Here's how the part is built. I have some questions about the finished solid (model axes, mm). Face numbers are marked on the shaded views. A direction names the side the tool comes from. Coordinates: 2 decimals unless noted, no trailing zeros. Write each loop counter-clockwise with the first axis right and the second up, starting at its lowest first coordinate (ties: lowest second). Pieces come first, ordered by that corner, then holes. Notation, with made-up numbers: (83.25, 34.25) -> (101.25, 34.25) arc R19 ccw to (101.25, 67.25) -> close; hole circle Ø10 at (-33.75, 5). An arc over 180 degrees is marked (long way). Use a Markdown table: item, result. Add a question column.
Item 1: If I drill on line 1 along Z through (x, y) = (6, -0.75); line 2 along Y through (x, z) = (-16.5, -3.5); line 3 along Y through (x, z) = (-10, -4.25), over which ranges is the centre line in solid material (lowest first)? Write a range as from..to.
Item 2: If we mould it in two halves opening along Z, with no side actions, what happens to the marked faces 1, 2 and 3? For each: pulls with the +Z half, pulls with the -Z half, needs draft (parallel to the pull), parting line crosses it, or undercut.
Item 3: Imagine slicing it at C-C, the plane x = 8.89. Write out the boundary of the cut face in (y, z).
Item 4: On a 3-axis mill with a long thin cutter (end or side, diameter ignored), from which of +Z, -Z, +X, -X, +Y, -Y can I reach the whole of each face in a straight line? I mean the marked faces 4, 5, 6, 7 and 8. Say none if no direction works.
Item 5: Imagine slicing it at D-D, the plane y = 8.75. Write out the boundary of the cut face in (x, z) (3 decimals), and give its area (3 significant figures).
Item 6: Will these pins go through, and if not, where does the flat tip stop? pin 1 Ø2 at (x, z) = (-2.5, 6.5) entering from -Y; pin 2 Ø5 at (y, z) = (6.5, -0.5) entering from +X; pin 3 Ø4 at (x, z) = (-3, -2) entering from -Y.
Item 7: Imagine slicing it at A-A, the plane y = 4.75. Write out the boundary of the cut face in (x, z) (3 decimals), and give its area (3 significant figures).
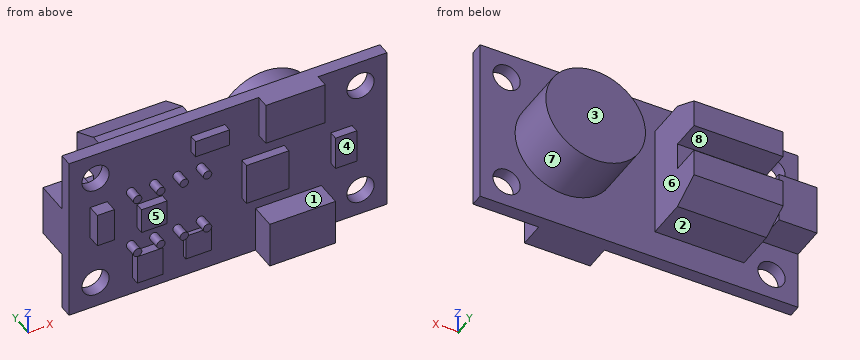
```python
from build123d import *

# Parameters (mm, degrees)
SKETCH1_W               = 38.1
SKETCH1_H               = 20.32
BOSS_EXTRUDE1_DEPTH     = 1.524
F_4_CLEARANCE_HOLE1_D   = 3.2639
SKETCH4_W               = 4.572
SKETCH4_H               = 6.096
BOSS_EXTRUDE2_DEPTH     = 4.064
SKETCH5_R               = 5.969
BOSS_EXTRUDE3_DEPTH     = 6.604
SKETCH6_W               = 10.668
SKETCH6_H               = 13.462
BOSS_EXTRUDE4_DEPTH     = 4.826
BOSS_EXTRUDE5_DEPTH     = 10.668
SKETCH8_W               = 7.874
SKETCH8_H               = 5.588
BOSS_EXTRUDE6_DEPTH     = 3.048
SKETCH9_W               = 7.112
SKETCH9_H               = 5.08
BOSS_EXTRUDE7_DEPTH     = 1.524
SKETCH10_W              = 2.54
SKETCH10_H              = 4.064
BOSS_EXTRUDE8_DEPTH     = 1.016
SKETCH11_W              = 5.08
SKETCH11_H              = 5.08
BOSS_EXTRUDE9_DEPTH     = 1.016
SKETCH12_W              = 4.064
SKETCH12_H              = 2.032
BOSS_EXTRUDE10_DEPTH    = 1.016
SKETCH13_W              = 3.048
SKETCH13_H              = 3.048
BOSS_EXTRUDE11_DEPTH    = 0.508
SKETCH14_W              = 3.048
SKETCH14_H              = 3.556
BOSS_EXTRUDE12_DEPTH    = 1.016
SKETCH15_W              = 2.032
SKETCH15_H              = 4.064
BOSS_EXTRUDE13_DEPTH    = 1.524
SKETCH16_W              = 3.048
SKETCH16_H              = 3.048
BOSS_EXTRUDE14_DEPTH    = 1.016
SKETCH17_R              = 0.508
BOSS_EXTRUDE15_DEPTH    = 1.524
LPATTERN1_COUNT         = 4
LPATTERN1_PITCH         = 2.794
MIRROR1_COPY_1_SKETCH_R = 0.508
MIRROR1_COPY_1_DEPTH    = 1.524
MIRROR1_COPY_2_SKETCH_R = 0.508
MIRROR1_COPY_2_DEPTH    = 1.524
MIRROR1_COPY_3_SKETCH_R = 0.508
MIRROR1_COPY_3_DEPTH    = 1.524


with BuildPart() as part:
    # Sketch1 → Boss-Extrude1 (new body)
    with BuildSketch(Plane(origin=(0, 0, 0), x_dir=(1, 0, 0), z_dir=(0, 1, 0))):
        Rectangle(SKETCH1_W, SKETCH1_H)
    extrude(amount=BOSS_EXTRUDE1_DEPTH)

    # #4 Clearance Hole1 (through all)
    with Locations(Plane(origin=(0, 1.524, 0), x_dir=(1, 0, 0), z_dir=(0, 1, 0))):
        with Locations((-15.875, 6.985), (15.875, -6.985), (-15.875, -6.985), (15.875, 6.985)):
            Hole(F_4_CLEARANCE_HOLE1_D / 2)

    # Sketch4 → Boss-Extrude2 (add)
    with BuildSketch(Plane(origin=(0, 1.524, 0), x_dir=(1, 0, 0), z_dir=(0, 1, 0))):
        with Locations((-16.764, 0)):
            Rectangle(SKETCH4_W, SKETCH4_H)
    extrude(amount=BOSS_EXTRUDE2_DEPTH)

    # Sketch5 → Boss-Extrude3 (add)
    with BuildSketch(Plane(origin=(0, 1.524, 0), x_dir=(1, 0, 0), z_dir=(0, 1, 0))):
        with Locations((8.89, 0)):
            Circle(SKETCH5_R)
    extrude(amount=BOSS_EXTRUDE3_DEPTH)

    # Sketch6 → Boss-Extrude4 (add)
    with BuildSketch(Plane(origin=(0, 1.524, 0), x_dir=(1, 0, 0), z_dir=(0, 1, 0))):
        with Locations((-7.239, 0)):
            Rectangle(SKETCH6_W, SKETCH6_H)
    extrude(amount=BOSS_EXTRUDE4_DEPTH)

    # Sketch7 → Boss-Extrude5 (add)
    with BuildSketch(Plane.ZY.offset(12.573)):
        Polygon((-6.731, 6.35), (-4.953, 9.906), (-1.651, 9.906), (-1.651, 6.35), align=None)
        Polygon((6.731, 6.35), (4.953, 9.906), (1.651, 9.906), (1.651, 6.35), align=None)
    extrude(amount=-BOSS_EXTRUDE5_DEPTH)

    # Sketch8 → Boss-Extrude6 (add)
    with BuildSketch(Plane.XZ):
        with Locations((7.239, -7.366)):
            Rectangle(SKETCH8_W, SKETCH8_H)
    extrude(amount=BOSS_EXTRUDE6_DEPTH)

    # Sketch9 → Boss-Extrude7 (add)
    with BuildSketch(Plane.XZ):
        with Locations((7.239, 7.62)):
            Rectangle(SKETCH9_W, SKETCH9_H)
    extrude(amount=BOSS_EXTRUDE7_DEPTH)

    # Sketch10 → Boss-Extrude8 (add)
    with BuildSketch(Plane.XZ):
        with Locations((13.589, 0)):
            Rectangle(SKETCH10_W, SKETCH10_H)
    extrude(amount=BOSS_EXTRUDE8_DEPTH)

    # Sketch11 → Boss-Extrude9 (add)
    with BuildSketch(Plane.XZ):
        with Locations((4.191, 0)):
            Rectangle(SKETCH11_W, SKETCH11_H)
    extrude(amount=BOSS_EXTRUDE9_DEPTH)

    # Sketch12 → Boss-Extrude10 (add)
    with BuildSketch(Plane.XZ):
        with Locations((-2.413, 7.112)):
            Rectangle(SKETCH12_W, SKETCH12_H)
    extrude(amount=BOSS_EXTRUDE10_DEPTH)

    # Sketch13 → Boss-Extrude11 (add)
    with BuildSketch(Plane.XZ):
        with Locations((-3.81, -6.096)):
            Rectangle(SKETCH13_W, SKETCH13_H)
    extrude(amount=BOSS_EXTRUDE11_DEPTH)

    # Sketch14 → Boss-Extrude12 (add)
    with BuildSketch(Plane.XZ):
        with Locations((-9.906, -6.35)):
            Rectangle(SKETCH14_W, SKETCH14_H)
    extrude(amount=BOSS_EXTRUDE12_DEPTH)

    # Sketch15 → Boss-Extrude13 (add)
    with BuildSketch(Plane.XZ):
        with Locations((-15.494, 1.27)):
            Rectangle(SKETCH15_W, SKETCH15_H)
    extrude(amount=BOSS_EXTRUDE13_DEPTH)

    # Sketch16 → Boss-Extrude14 (add)
    with BuildSketch(Plane.XZ):
        with Locations((-9.398, 0)):
            Rectangle(SKETCH16_W, SKETCH16_H)
    extrude(amount=BOSS_EXTRUDE14_DEPTH)

    # Sketch17 → Boss-Extrude15 (add)
    with BuildSketch(Plane.XZ):
        with Locations((-11.684, -3.556)):
            Circle(SKETCH17_R)
    boss_extrude15 = extrude(amount=BOSS_EXTRUDE15_DEPTH)

    # LPattern1: Boss-Extrude15 ×4
    with Locations(*[(i * LPATTERN1_PITCH, 0, 0) for i in range(1, LPATTERN1_COUNT)]):
        add(boss_extrude15)

    # Mirror1: Boss-Extrude15 across plane
    add(boss_extrude15.mirror(Plane.XY))

    # Mirror1 copy 1 sketch → Mirror1 copy 1 (add)
    with BuildSketch(Plane(origin=(2.794, 0, 0), x_dir=(1, 0, 0), z_dir=(0, -1, 0))):
        with Locations((-11.684, 3.556)):
            Circle(MIRROR1_COPY_1_SKETCH_R)
    extrude(amount=MIRROR1_COPY_1_DEPTH)

    # Mirror1 copy 2 sketch → Mirror1 copy 2 (add)
    with BuildSketch(Plane(origin=(5.588, 0, 0), x_dir=(1, 0, 0), z_dir=(0, -1, 0))):
        with Locations((-11.684, 3.556)):
            Circle(MIRROR1_COPY_2_SKETCH_R)
    extrude(amount=MIRROR1_COPY_2_DEPTH)

    # Mirror1 copy 3 sketch → Mirror1 copy 3 (add)
    with BuildSketch(Plane(origin=(8.382, 0, 0), x_dir=(1, 0, 0), z_dir=(0, -1, 0))):
        with Locations((-11.684, 3.556)):
            Circle(MIRROR1_COPY_3_SKETCH_R)
    extrude(amount=MIRROR1_COPY_3_DEPTH)


solid = part.part
```
Ans:
| question | item | result |
|---|---|---|
| 1 | line 1 | z = -10.16..-4.57, -2.54..2.54, 5.08..10.16 |
| 1 | line 2 | y = 0..1.52 |
| 1 | line 3 | y = 0..9.91 |
| 2 | face 1 | undercut |
| 2 | face 2 | pulls with the -Z half |
| 2 | face 3 | needs draft |
| 3 | outline | (-3.05, -10.16) -> (1.52, -10.16) -> (1.52, -5.97) -> (8.13, -5.97) -> (8.13, 5.97) -> (1.52, 5.97) -> (1.52, 10.16) -> (-1.52, 10.16) -> (-1.52, 5.08) -> (0, 5.08) -> (0, -4.57) -> (-3.05, -4.57) -> close |
| 4 | face 4 | +Z, -Z, +X, -Y |
| 4 | face 5 | +X, -Y |
| 4 | face 6 | +Z, -Z, +Y |
| 4 | face 7 | +Y |
| 4 | face 8 | -X, +Y |
| 5 | outline | (-12.573, -5.531) -> (-1.905, -5.531) -> (-1.905, -1.651) -> (-12.573, -1.651) -> close; (-12.573, 1.651) -> (-1.905, 1.651) -> (-1.905, 5.531) -> (-12.573, 5.531) -> close |
| 5 | area | 82.8 mm^2 |
| 6 | pin 1 | stops at y = -1.02 |
| 6 | pin 2 | stops at x = 14.86 |
| 6 | pin 3 | stops at y = -1.52 |
| 7 | outline | (-19.05, -3.048) -> (-14.478, -3.048) -> (-14.478, 3.048) -> (-19.05, 3.048) -> close; (-12.573, -6.731) -> (-1.905, -6.731) -> (-1.905, 6.731) -> (-12.573, 6.731) -> close; circle Ø11.938 at (8.89, 0) |
| 7 | area | 283 mm^2 |
